CAD build for the part. Positions are in the model's coordinates, mm. Face numbers are marked on the shaded views. A direction names the side the tool comes from. Round coordinates to 2 decimals unless told otherwise and drop trailing zeros. Write each loop counter-clockwise with the first axis right and the second up, starting at its lowest first coordinate (ties: lowest second). Pieces come first, ordered by that corner, then holes. Notation, with made-up numbers: (40.25, 74.25) - (94.25, 74.25) arc R27 cw to (94.25, 104.25) - close; hole circle Ø7 at (89.5, 32.5). An arc over 180 degrees is marked (long way). Put each result on its own line as item: value. Start each with the question number.
Item 1: Cut at C-C (x = -22). Give the cut face in (y, z).
Item 2: Drill centre lines: line 1 (X direction, y = 144.5, z = 15); line 2 (Z direction, x = -16.75, y = 158.5); line 3 (Z direction, x = -11, y = 148). Where is each one in solid material? Low to high. Write a range as from..to.
Item 3: Pin check, flat tips, straight feed: pin 1 Ø6 at (y, z) = (135.5, 15) entering from -X; pin 2 Ø5 at (x, z) = (-25, 4) entering from -Y; pin 3 Ø3 at (x, y) = (-18, 157) entering from +Z. Stop position of each tip, or through.
Item 4: Cut at D-D (z = 5.75). Give the cut face in (x, y).
Item 5: Mould opens along X. For the marked faces 1, 2 and 3 say: released by +X, released by -X, zero draft, split by the parting line, or undercut.
Item 6: Cut at B-B (y = 156.75). Give the cut face in (x, z), and give its area (3 significant figures).
Item 7: 3-axis set-ups, long thin cutter, end or side, ignore diameter. For the marked faces 4, 5 and 6: which of +Z, -Z, +X, -X, +Y, -Y reach the whole face in a straight line?
```python
from build123d import *
from OCP.BRepFilletAPI import BRepFilletAPI_MakeChamfer

# Parameters (mm, degrees)
SKETCH1_W                       = 16.5
SKETCH1_H                       = 33
BOSS_EXTRUDE1_DEPTH             = 20
FILLET1_R                       = 8.25
CHAMFER1_SIZE                   = 8.25
CHAMFER1_SIZE_2                 = 4.763139721
SKETCH2_W                       = 16.5
SKETCH2_H                       = 33
SKETCH2_R                       = 5.85
SKETCH2_R_2                     = 5.05
CUT_EXTRUDE1_DEPTH              = 10
FILLET2_R                       = 5
SKETCH4_R                       = 5.1
BOSS_EXTRUDE2_DEPTH             = 7.3
SCHNITT_LINEAR_AUSTRAGEN1_DEPTH = 9


with BuildPart() as part:
    # Sketch1 → Boss-Extrude1 (new body)
    with BuildSketch(Plane.XY):
        with Locations((-18.614437814, 148.5)):
            Rectangle(SKETCH1_W, SKETCH1_H)
    extrude(amount=BOSS_EXTRUDE1_DEPTH)

    # Fillet1
    fillet1_edges = [part.edges().sort_by_distance(p)[0] for p in [
        (-26.864437814, 132, 10),
        (-10.364437814, 132, 10),
    ]]
    fillet(fillet1_edges, radius=FILLET1_R - 0.0001)  # a hair under: the kernel refuses the full size

    # Chamfer1
    chamfer1_edges_1 = [part.edges().sort_by_distance(p)[0] for p in [
        (-26.864437814, 165, 10),
    ]]
    chamfer1_side_1 = [part.faces().sort_by_distance(p)[0] for p in [
        (-26.769175019, 165, 10),
    ]]
    chamfer1_edges_2 = [part.edges().sort_by_distance(p)[0] for p in [
        (-10.364437814, 165, 10),
    ]]
    chamfer1_side_2 = [part.faces().sort_by_distance(p)[0] for p in [
        (-10.364437814, 164.904737206, 10),
    ]]
    chamfer1 = BRepFilletAPI_MakeChamfer(part.part.solid().wrapped)
    for e in chamfer1_edges_1:
        chamfer1.Add(CHAMFER1_SIZE - 0.0001, CHAMFER1_SIZE_2 - 0.0001, e.wrapped, chamfer1_side_1[0].wrapped)
    for e in chamfer1_edges_2:
        chamfer1.Add(CHAMFER1_SIZE_2 - 0.0001, CHAMFER1_SIZE - 0.0001, e.wrapped, chamfer1_side_2[0].wrapped)
    add(Compound.cast(chamfer1.Shape()), mode=Mode.REPLACE)  # a hair under: the kernel refuses the full size

    # Sketch2 → Cut-Extrude1 (cut)
    # profile 1 of 3: a face of its own
    with BuildSketch(Plane(origin=(0, 0, 0), x_dir=(-1, 0, 0), z_dir=(0, 0, -1))):
        with Locations((18.614437814, 148.5)):
            Rectangle(SKETCH2_W, SKETCH2_H)
        with Locations((18.614437814, 156.75)):
            Circle(SKETCH2_R, mode=Mode.SUBTRACT)
        with Locations((18.614437814, 140.25)):
            Circle(SKETCH2_R, mode=Mode.SUBTRACT)
    # profile 2 of 3: a face of its own
    with BuildSketch(Plane(origin=(0, 0, 0), x_dir=(-1, 0, 0), z_dir=(0, 0, -1))):
        with Locations((18.614437814, 140.25)):
            Circle(SKETCH2_R_2)
    # profile 3 of 3: a face of its own
    with BuildSketch(Plane(origin=(0, 0, 0), x_dir=(-1, 0, 0), z_dir=(0, 0, -1))):
        with Locations((18.614437814, 156.75)):
            Circle(SKETCH2_R_2)
    extrude(amount=-CUT_EXTRUDE1_DEPTH, mode=Mode.SUBTRACT)

    # Fillet2
    fillet2_edges = [part.edges().sort_by_distance(p)[0] for p in [
        (-26.864437814, 160.236960279, 15),
        (-10.364437814, 160.236960279, 15),
    ]]
    fillet(fillet2_edges, radius=FILLET2_R)

    # Sketch4 → Boss-Extrude2 (add)
    with BuildSketch(Plane(origin=(0, 0, 10), x_dir=(-1, 0, 0), z_dir=(0, 0, -1))):
        with Locations((18.614437814, 156.75)):
            Circle(SKETCH4_R)
        with Locations((18.614437814, 140.25)):
            Circle(SKETCH4_R)
    extrude(amount=BOSS_EXTRUDE2_DEPTH)

    # Skizze1 → Schnitt-Linear austragen1 (cut)
    with BuildSketch(Plane.XY.offset(20)):
        with BuildLine():
            Line((-12.364437814, 140.25), (-12.364437814, 157.350108933))
            ThreePointArc((-12.364437814, 157.350108933), (-12.766361602, 158.850108933), (-13.864437814, 159.948185145))
            Line((-13.864437814, 159.948185145), (-18.614437814, 162.690598923))
            Line((-18.614437814, 162.690598923), (-23.364437814, 159.948185145))
            ThreePointArc((-23.364437814, 159.948185145), (-24.462514025, 158.850108933), (-24.864437814, 157.350108933))
            Line((-24.864437814, 157.350108933), (-24.864437814, 140.25))
            ThreePointArc((-24.864437814, 140.25), (-23.033855196, 135.830582618), (-18.614437814, 134))
            ThreePointArc((-18.614437814, 134), (-14.195020431, 135.830582618), (-12.364437814, 140.25))
        make_face()
    extrude(amount=-SCHNITT_LINEAR_AUSTRAGEN1_DEPTH, mode=Mode.SUBTRACT)


solid = part.part
```
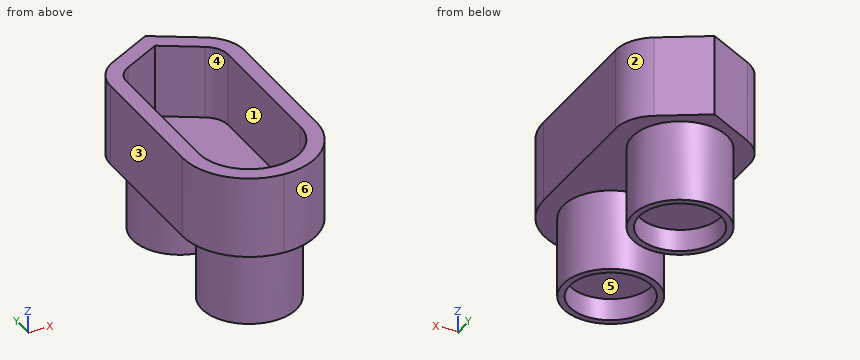
Output values:
1. outline: (132.73, 10) - (135.48, 10) - (135.48, 0) - (136.5, 0) - (136.5, 2.7) - (144, 2.7) - (144, 0) - (145.02, 0) - (145.02, 10) - (151.98, 10) - (151.98, 0) - (153, 0) - (153, 2.7) - (160.5, 2.7) - (160.5, 0) - (161.52, 0) - (161.52, 10) - (163.05, 10) - (163.05, 20) - (160.74, 20) - (160.74, 11) - (135, 11) - (135, 20) - (132.73, 20) - close
2. line 1: -26.86..-24.86, -12.36..-10.36
2. line 2: 2.7..11
2. line 3: 10..20
3. pin 1: x = -26.68
3. pin 2: y = 135.88
3. pin 3: z = 11
4. outline: circle Ø11.7 at (-18.61, 140.25); circle Ø11.7 at (-18.61, 156.75)
5. face 1: undercut
5. face 2: released by +X
5. face 3: released by -X
6. outline: (-26.86, 10) - (-24.46, 10) - (-24.46, 0) - (-23.66, 0) - (-23.66, 2.7) - (-13.56, 2.7) - (-13.56, 0) - (-12.76, 0) - (-12.76, 10) - (-10.36, 10) - (-10.36, 20) - (-12.36, 20) - (-12.36, 11) - (-24.86, 11) - (-24.86, 20) - (-26.86, 20) - close
6. area: 142 mm2
7. face 4: +Z
7. face 5: -Z
7. face 6: +Z, -Z, +X, -Y
